Work out the finished part from the listing and answer in its coordinate system (mm). Face numbers are marked on the shaded views. A direction names the side the tool comes from. Coordinates: 2 decimals unless noted, no trailing zeros. Order: outer loops, then holes, each group sorted by start corner. A loop starts at its lowest first (then second) coordinate and runs counter-clockwise, first axis right, second up. Notation, with made-up numbers: M 41.25,17 L 63.25,17 A17 ccw 63.25,44 Z; hole C 81.5,-29 d8. An arc over 180 degrees is marked long. Use a Markdown table: item, result.
Autodesk Inventor part; units mm, degrees
ref_plane "YZ Plane" through (0, 0, 0) normal (1, 0, 0) x (0, 1, 0)
ref_plane "XZ Plane" through (0, 0, 0) normal (0, 1, 0) x (-1, 0, 0)
ref_plane "XY Plane" through (0, 0, 0) normal (0, 0, 1) x (1, 0, 0)
sketch "Skizze1" plane through (0, 0, 0) normal (0, 0, 1) x (1, 0, 0)
  line L0 (-25, 15) -> (25, 15)
  line L1 (25, 15) -> (25, -15)
  line L2 (25, -15) -> (-25, -15)
  line L3 (-25, -15) -> (-25, 15)
  line L4 (-25, 15) -> (25, -15) construction
  line L5 (25, 15) -> (-25, -15) construction
  point P0 (0, 0)
  dimension "d0" = 50
  dimension "d1" = 30
extrude "Extrusion1" add sketch "Skizze1" along normal mid plane 10
sketch "Skizze3" plane through (0, 0, 5) normal (0, 0, 1) x (1, 0, 0)
  line L0 (-35, 0) -> (35, 0)
  line L1 (25, 15) -> (-25, 15)
  line L2 (0, -21) -> (0, 21)
  line L3 (0, 21) -> (0, -21)
  point P0 (0, 0)
  point P1 (0, -10)
  point P2 (15, 5)
  dimension "d6" = 25
  dimension "d16" = 10
  dimension "d31" = 15
hole "Bohrung1" at (0, -10, 5) direction (0, 0, -1) diameter 4.917 end through all
hole "Bohrung2" at (15, 5, 5) direction (0, 0, -1) diameter 6.6 end through all counterbore diameter 11 counterbore depth 6.4
mirror "Spiegeln1" about plane through (0, 0, 0) normal (1, 0, 0) of "Bohrung2"
equation "\"d0\" = Länge_Vertikalbegrenzung"
equation "\"d1\" = Breite_Vertikalbegrenzung"
equation "\"d2\" = Tiefe_Vertikalbegrenzung"
equation "\"Länge_Vertikalbegrenzung\" = 50"
equation "\"Breite_Vertikalbegrenzung\" = 30"
equation "\"Tiefe_Vertikalbegrenzung\" = 10"
equation "\"Abstand_Bohrung_Madenschraube\" = 25"
equation "\"Abstand_Bohrungen_x\" = 15"
equation "\"Abstand_Bohrungen_y\" = 10"
properties part number "JH_Positionierungseinheit_Vertikalbegrenzung_int"
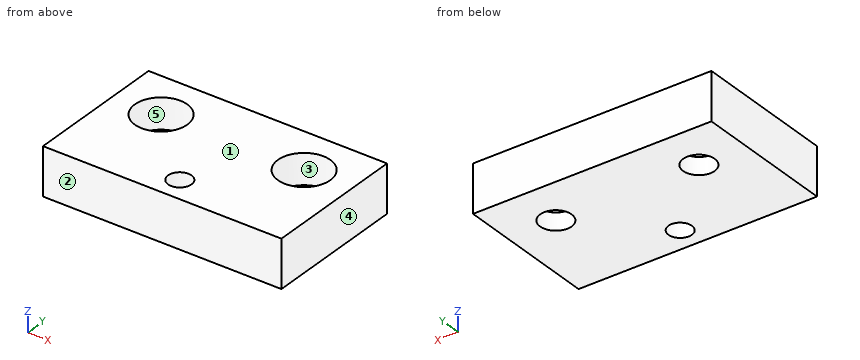
(1) Which of the six approach directions +Z, -Z, +X, -X, +Y, -Y give full straight-line access (tool end or side, diameter ignored) to the marked faces 4 and 5?
Conclusion:
| item | result |
|---|---|
| face 4 | +Z, -Z, +X, +Y, -Y |
| face 5 | +Z |
(2) A cutting plane is placed at D-D (y = -10). Determine the outline of the cut face in (x, z).
Conclusion:
| item | result |
|---|---|
| outline | M -25,-5 L -2.46,-5 L -2.46,5 L -25,5 Z; M 2.46,-5 L 25,-5 L 25,5 L 2.46,5 Z |
(3) A cutting plane is placed at A-A (x = -15). Determine the outline of the cut face in (y, z).
Conclusion:
| item | result |
|---|---|
| outline | M -15,-5 L 1.7,-5 L 1.7,-1.4 L -0.5,-1.4 L -0.5,5 L -15,5 Z; M 8.3,-5 L 15,-5 L 15,5 L 10.5,5 L 10.5,-1.4 L 8.3,-1.4 Z |
(4) Given P1, Ø9, axis at x = 15, y = 5, coming from the +Z side, flat-ended and moving along its own axis, determine where the tip first touches the part or whether it passes through.
Conclusion:
| item | result |
|---|---|
| P1 | z = -1.4 |
(5) Straight lines are drawn through the part: L1, parallel to X at y = 5, z = -2.55; L2, parallel to X at y = 4.75, z = 2.75; L3, parallel to Y at x = -15, z = -2.75. For each, find the intervals that lie inside material, in ascending order.
Conclusion:
| item | result |
|---|---|
| L1 | -25 to -18.3, -11.7 to 11.7, 18.3 to 25 |
| L2 | -25 to -20.49, -9.51 to 9.51, 20.49 to 25 |
| L3 | -15 to 1.7, 8.3 to 15 |
(6) A cutting plane is placed at C-C (z = 0.25). Determine the outline of the cut face in (x, y).
Conclusion:
| item | result |
|---|---|
| outline | M -25,-15 L 25,-15 L 25,15 L -25,15 Z; hole C -15,5 d11; hole C 0,-10 d4.92; hole C 15,5 d11 |
(7) Determine the mould class of the marked faces 1, 2 and 3 for opening direction Y: pulls with the +Y half, pulls with the -Y half, needs draft (parallel to the pull), parting line crosses it, or undercut.
Conclusion:
| item | result |
|---|---|
| face 1 | needs draft |
| face 2 | pulls with the -Y half |
| face 3 | undercut |
(8) A cutting plane is placed at B-B (y = 5). Determine the outline of the cut face in (x, z).
Conclusion:
| item | result |
|---|---|
| outline | M -25,-5 L -18.3,-5 L -18.3,-1.4 L -20.5,-1.4 L -20.5,5 L -25,5 Z; M -11.7,-5 L 11.7,-5 L 11.7,-1.4 L 9.5,-1.4 L 9.5,5 L -9.5,5 L -9.5,-1.4 L -11.7,-1.4 Z; M 18.3,-5 L 25,-5 L 25,5 L 20.5,5 L 20.5,-1.4 L 18.3,-1.4 Z |
